The listing builds one solid part. Answer for the finished solid, in the listing's coordinates (mm). A direction names the side the tool comes from. Round coordinates to 2 decimals unless told otherwise and drop trailing zeros. Write each loop counter-clockwise with the first axis right and the second up, starting at its lowest first coordinate (ties: lowest second). Pieces come first, ordered by that corner, then holes.
Item 1: Find section B-B on z = 1.55. Give the number of separate pieces and of enclosed holes in the cut face, then the cut area to 3 significant figures.
Item 2: A tool of negligible diameter and unlimited length cuts with its end or side. For faces 5 (the face through (-76, -55, 2)), 6 (the face through (23.234, -63, 2)), from which of +Z, -Z, +X, -X, +Y, -Y can it reach the whole face along a straight path? Write none if from no direction.
Item 3: Find section A-A on x = -63.02. Give the vertices of the cut face in (y, z), then the cut area to 3 significant figures.
Item 4: Each of these flat-tipped pins is pushed along its axis until it touches: pin 1 (2 mm diameter, centred on y = -62.5, z = 1.5, fed in from -X); pin 2 (2.5 mm diameter, centred on x = -56.67, y = 11.93, fed in from +Z); pin 3 (1.5 mm diameter, centred on x = -44, z = 3, fed in from -Y); pin 4 (1.2 mm diameter, centred on y = -62.5, z = 1.5, fed in from +X). Where does it stop, or does it pass through?
Item 5: For a pull along X with two mould halves and no side action, classify faces 1 (the face through (17.826, 9.978, 2.028)), 2 (the face through (-80.65, 61.99, 2.03)), 3 (the face through (-76, 55, 2)), 4 (the face through (-1, 65, 2)) as +X half, -X half, draft (parallel to the pull), parting line (faces both ways), or undercut.
Item 6: Find the intervals of material crossed by probe 1 along Y at (x, z) = (73.5, 1.6); probe 2 along Y at (x, z) = (-48, 2.45); probe 3 along Y at (x, z) = (-56.67, 2.4), in increasing order.
Item 7: Find section C-C on x = 32. Give the vertices of the cut face in (y, z), then the cut area to 3 significant figures.
```python
from build123d import *

# Parameters (mm, degrees)
SKETCH1_W           = 167
SKETCH1_H           = 130
BOSS_EXTRUDE1_DEPTH = 4
FILLET1_R           = 10
FILLET2_R           = 10
SKETCH5_R           = 2.5
CUT_EXTRUDE4_DEPTH  = 70
SKETCH6_W           = 30
SKETCH6_H           = 5
CUT_EXTRUDE5_DEPTH  = 10
SKETCH10_R          = 2
CUT_EXTRUDE9_DEPTH  = 106.892634305
SKETCH11_R          = 2
CUT_EXTRUDE10_DEPTH = 106.892634305


with BuildPart() as part:
    # Sketch1 → Boss-Extrude1 (new body)
    with BuildSketch(Plane.XY):
        Rectangle(SKETCH1_W, SKETCH1_H)
    extrude(amount=BOSS_EXTRUDE1_DEPTH)

    # Fillet1
    fillet1_edges = [part.edges().sort_by_distance(p)[0] for p in [
        (-83.5, -65, 2),
        (-83.5, 65, 2),
    ]]
    fillet(fillet1_edges, radius=FILLET1_R)

    # Fillet2
    fillet2_edges = [part.edges().sort_by_distance(p)[0] for p in [
        (83.5, -65, 2),
        (83.5, 65, 2),
    ]]
    fillet(fillet2_edges, radius=FILLET2_R)

    # Sketch5 → Cut-Extrude4 (cut)
    with BuildSketch(Plane.XY.offset(4)):
        with Locations((-73.5, 55)):
            Circle(SKETCH5_R)
        with Locations((73.5, 55)):
            Circle(SKETCH5_R)
        with Locations((-73.5, -55)):
            Circle(SKETCH5_R)
        with Locations((73.5, -55)):
            Circle(SKETCH5_R)
    extrude(amount=-CUT_EXTRUDE4_DEPTH, mode=Mode.SUBTRACT)

    # Sketch6 → Cut-Extrude5 (cut)
    with BuildSketch(Plane.XY.offset(4)):
        with Locations((-38.233797414, -62.5)):
            Rectangle(SKETCH6_W, SKETCH6_H)
        with Locations((38.233797414, -62.5)):
            Rectangle(SKETCH6_W, SKETCH6_H)
    extrude(amount=-CUT_EXTRUDE5_DEPTH, mode=Mode.SUBTRACT)

    # Sketch10 → Cut-Extrude9 (cut, through all)
    with BuildSketch(Plane.XY.offset(4)):
        with Locations((-48, -1.106245372)):
            Circle(SKETCH10_R)
        with Locations((10, -50.106245372)):
            Circle(SKETCH10_R)
        with Locations((-48, -50.106245372)):
            Circle(SKETCH10_R)
        with Locations((10, -1.106245372)):
            Circle(SKETCH10_R)
    extrude(amount=-CUT_EXTRUDE9_DEPTH, mode=Mode.SUBTRACT)

    # Sketch11 → Cut-Extrude10 (cut, through all)
    with BuildSketch(Plane.XY.offset(4)):
        with Locations((-63.02, 60.190179321)):
            Circle(SKETCH11_R)
        with Locations((-32.54, 55.110179321)):
            Circle(SKETCH11_R)
        with Locations((-32.54, 27.170179321)):
            Circle(SKETCH11_R)
        with Locations((19.53, 60.190179321)):
            Circle(SKETCH11_R)
        with Locations((18.26, 11.930179321)):
            Circle(SKETCH11_R)
        with Locations((-56.67, 11.930179321)):
            Circle(SKETCH11_R)
    extrude(amount=-CUT_EXTRUDE10_DEPTH, mode=Mode.SUBTRACT)


solid = part.part
```
Check values:
1. separate pieces: 1
1. enclosed holes: 14
1. area: 21,100 mm2
2. face 5: +Z, -Z
2. face 6: +Z, -Z, -Y
3. outline: (-65, 0) - (58.19, 0) - (58.19, 4) - (-65, 4) - close; (62.19, 0) - (65, 0) - (65, 4) - (62.19, 4) - close
3. area: 504 mm2
4. pin 1: stops at x = -81.1
4. pin 2: passes through
4. pin 3: stops at y = -60
4. pin 4: stops at x = 80.74
5. face 1: undercut
5. face 2: -X half
5. face 3: undercut
5. face 4: draft
6. probe 1: y = -65 to -57.5, -52.5 to 52.5, 57.5 to 65
6. probe 2: y = -60 to -52.11, -48.11 to -3.11, 0.89 to 65
6. probe 3: y = -65 to 9.93, 13.93 to 65
7. outline: (-60, 0) - (65, 0) - (65, 4) - (-60, 4) - close
7. area: 500 mm2
